For this review, take the finished solid that the model builds, in its own axes (mm). A direction names the side the tool comes from. Give positions to 0.01 mm unless a question says otherwise; leave off trailing zeros. Loops run counter-clockwise (first coordinate to the right, second up) from the corner with the lowest first, then second, coordinate; pieces in that order, holes last.
Autodesk Fusion 360 part; units mm, degrees
sketch "スケッチ1" plane through (0, 0, 0) normal (0, 0, 1) x (1, 0, 0)
  line L0 (-9.5, 140) -> (-80.5, 140)
  line L1 (-80.5, 140) -> (-80.5, -140)
  line L2 (-80.5, -140) -> (-9.5, -140)
  line L3 (80.5, -80) -> (80.5, 130)
  line L4 (74.75, 130) -> (-80.5, -140) construction
  line L5 (-9.5, 140) -> (-9.5, 130)
  line L6 (-9.5, 130) -> (80.5, 130)
  line L7 (-80.5, -140) -> (-9.5, -140) construction
  line L8 (-9.5, -140) -> (80.5, -100)
  line L9 (80.5, -100) -> (-9.5, -100)
  line L10 (-9.5, -100) -> (-9.5, -80)
  line L11 (-9.5, -80) -> (80.5, -80)
  line L12 (-80.5, 140) -> (46, -80) construction
  line L13 (57.5, -100) -> (62.1814, -108.1416) construction
  dimension "d2" = 280
  dimension "d5" = 71
  dimension "d7" = 90
  dimension "d8" = 20
extrude "押し出し1" add sketch "スケッチ1" along normal blind 6
chamfer "面取り1" distance 25 angle 45 2 edges at (-80.5, -140, 3) (-80.5, 140, 3)
sketch "スケッチ2" plane through (0, 0, 6) normal (0, 0, 1) x (-1, 0, 0)
  line L0 (55.5, -140) -> (80.5, -115)
  line L1 (80.5, -115) -> (80.5, 115)
  line L2 (80.5, 115) -> (55.5, 140)
  line L3 (55.5, 140) -> (9.5, 140)
  line L4 (9.5, 140) -> (-80.5, 100)
  line L5 (-80.5, 100) -> (9.5, 100)
  line L6 (9.5, 100) -> (9.5, 80)
  line L7 (9.5, 80) -> (-80.5, 80)
  line L8 (-80.5, 80) -> (-80.5, -130)
  line L9 (-80.5, -130) -> (9.5, -130)
  line L10 (9.5, -130) -> (9.5, -140)
  line L11 (9.5, -140) -> (55.5, -140)
  line L12 (-80.5, -130) -> (-40.5, -130) construction
  line L13 (-40.5, -130) -> (-40.5, -85) construction
  line L14 (-40.5, -85) -> (-80.5, -85) construction
  line L15 (-80.5, -85) -> (-80.5, -130) construction
  line L16 (-40.5, -85) -> (-40.5, -25) construction
  line L17 (-40.5, -25) -> (-40.5, 35) construction
  point P0 (-40.5, -85)
  point P1 (-40.5, -25)
  point P2 (-40.5, 35)
  dimension "d12" = 40
  dimension "d13" = 45
  dimension "d14" = 60
  dimension "d15" = 60
hole "穴1" at (40.5, 85, 6) at (40.5, 25, 6) at (40.5, -35, 6) direction (0, 0, -1) diameter 18 end through all
equation "d5 = 25 mm + 46 mm"
Item 1: Take a section at A-A on y = 25. Give the boundary of the cut face in (x, z).
Answer:
outline: (-80.5, 0) - (31.5, 0) - (31.5, 6) - (-80.5, 6) - close; (49.5, 0) - (80.5, 0) - (80.5, 6) - (49.5, 6) - close
Item 2: For L1, parallel to X at y = 25, z = 2.05; L2, parallel to Y at x = 40.5, z = 3.6; L3, parallel to Y at x = 64, z = 0.6, list the stretches that pass through material, from the lowest coordinate up.
Answer:
L1: x = -80.5 to 31.5, 49.5 to 80.5
L2: y = -117.78 to -100, -80 to -44, -26 to 16, 34 to 76, 94 to 130
L3: y = -107.33 to -100, -80 to 130
Item 3: Clearance check with flat-ended pins moving along their axes: pin 1 Ø2 at (x, z) = (52, 3) entering from -Y; pin 2 Ø2 at (x, z) = (4.5, 1.5) entering from -Y; pin 3 Ø1.8 at (x, z) = (26.5, 1.5) entering from -Y. State where each tip first meets the part, or that it passes through.
Answer:
pin 1: stops at y = -113.11
pin 2: stops at y = -134.22
pin 3: stops at y = -124.4
Item 4: Tool access review of faces 4 (the flat face through (-9.5, 135, 3)), 5 (the flat face through (36, -100, 3)), 6 (the flat face through (80.5, 24, 3)): name each direction out of +Z, -Z, +X, -X, +Y, -Y from which nothing blocks a thin tool from reaching the whole face with its end or side.
Answer:
face 4: +Z, -Z, +X, +Y
face 5: +Z, -Z, +X
face 6: +Z, -Z, +X, +Y, -Y
Item 5: Take a section at C-C on x = 16. Give the boundary of the cut face in (y, z), and give its area (3 significant figures).
Answer:
outline: (-128.67, 0) - (-100, 0) - (-100, 6) - (-128.67, 6) - close; (-80, 0) - (130, 0) - (130, 6) - (-80, 6) - close
area: 1,430 mm2
Item 6: Take a section at D-D on y = -123. Give the boundary of the cut face in (x, z).
Answer:
outline: (-72.5, 0) - (28.75, 0) - (28.75, 6) - (-72.5, 6) - close
Item 7: The part is to be moulded in two halves that separate along X. For faces 1 (the flat face through (-1, 2, 0)), 2 (the cylindrical face through (32.91, 20.16, 2.96)), 3 (the flat face through (-9.5, -90, 3)), say which applies: released by +X, released by -X, zero draft, split by the parting line, or undercut.
Answer:
face 1: zero draft
face 2: undercut
face 3: released by +X
Item 8: Take a section at B-B on z = 4.45. Give the boundary of the cut face in (x, y), and give its area (3 significant figures).
Answer:
outline: (-80.5, -115) - (-55.5, -140) - (-9.5, -140) - (80.5, -100) - (-9.5, -100) - (-9.5, -80) - (80.5, -80) - (80.5, 130) - (-9.5, 130) - (-9.5, 140) - (-55.5, 140) - (-80.5, 115) - close; hole circle Ø18 at (40.5, -35); hole circle Ø18 at (40.5, 25); hole circle Ø18 at (40.5, 85)
area: 39,200 mm2
